```python
from build123d import *

# Parameters (mm, degrees)
SKETCH1_W           = 127
SKETCH1_H           = 127
BOSS_EXTRUDE1_DEPTH = 12.7
CUT_EXTRUDE1_REACH  = 14.7
SKETCH2_R           = 51.5


with BuildPart() as part:
    # Sketch1 → Boss-Extrude1 (new body)
    with BuildSketch(Plane.XY):
        Rectangle(SKETCH1_W, SKETCH1_H)
    extrude(amount=BOSS_EXTRUDE1_DEPTH)

    # Sketch2 → Cut-Extrude1 (cut, up to next)
    with BuildSketch(Plane.XY.offset(12.7), mode=Mode.PRIVATE) as cut_extrude1_sk1:
        Circle(SKETCH2_R)
    cut_extrude1_tool1 = extrude(cut_extrude1_sk1.sketch, amount=-CUT_EXTRUDE1_REACH, mode=Mode.PRIVATE) & part.part
    add(cut_extrude1_tool1.solids().sort_by_distance((0, 0, 12.7))[0], mode=Mode.SUBTRACT)


solid = part.part
```
Part model, mm, in its own coordinate system. Round coordinates to 2 decimals unless told otherwise and drop trailing zeros. Write each loop counter-clockwise with the first axis right and the second up, starting at its lowest first coordinate (ties: lowest second). Pieces come first, ordered by that corner, then holes.
Item 1: Two-plate mould, pull along Y, no slides. Class faces 1 (the cylindrical face through (-11.164, -50.275, 6.439)), 2 (the flat face through (63.5, -1, 6)), 3 (the flat face through (-1, 63.5, 6)): +Y half, -Y half, draft (parallel to the pull), parting line (faces both ways), or undercut.
Results:
face 1: undercut
face 2: draft
face 3: +Y half
Item 2: Drop a flat-ended pin along its axis: pin 1 Ø5 at (x, y) = (30, -37.5) entering from -Z. Give the stop position or say it passes through.
Results:
pin 1: passes through
Item 3: Cut at C-C, the plane z = 10.75. Give the cut face in (x, y).
Results:
outline: (-63.5, -63.5) - (63.5, -63.5) - (63.5, 63.5) - (-63.5, 63.5) - close; hole circle Ø103 at (0, 0)
Item 4: Probe L1, parallel to Y at x = 0, z = 8; L2, parallel to Y at x = 15, z = 3.75; L3, parallel to X at y = 25, z = 2.25 (3 decimals). List the from-to ranges inside material, lowest first.
Results:
L1: y = -63.5 to -51.5, 51.5 to 63.5
L2: y = -63.5 to -49.27, 49.27 to 63.5
L3: x = -63.5 to -45.025, 45.025 to 63.5
Item 5: Cut at A-A, the plane x = 0. Give the cut face in (y, z), plus the area to 3 significant figures.
Results:
outline: (-63.5, 0) - (-51.5, 0) - (-51.5, 12.7) - (-63.5, 12.7) - close; (51.5, 0) - (63.5, 0) - (63.5, 12.7) - (51.5, 12.7) - close
area: 305 mm2
